Input: part model. Units: mm. Frame: model coordinates. A direction names the side the tool comes from. Give positions to 0.01 mm unless a question says otherwise; leave off trailing zeros. Loops run counter-clockwise (first coordinate to the right, second up) from the corner with the lowest first, then second, coordinate; pieces in that order, holes last. Notation, with made-up numbers: M 57.25,69 L 76.25,69 A32 ccw 76.25,100 Z; hole C 67.5,-7.75 d11. An arc over 180 degrees is marked long. Use a Markdown table: item, result. Add a question column.
Autodesk Inventor part; units mm, degrees
ref_plane "YZ Plane" through (0, 0, 0) normal (1, 0, 0) x (0, 1, 0)
ref_plane "XZ Plane" through (0, 0, 0) normal (0, 1, 0) x (-1, 0, 0)
ref_plane "XY Plane" through (0, 0, 0) normal (0, 0, 1) x (1, 0, 0)
sketch "Szkic1" plane through (0, 0, 0) normal (0, 1, 0) x (-1, 0, 0)
  line L0 (0, 0) -> (25, 0)
  line L1 (25, 0) -> (25, -25)
  line L2 (25, -25) -> (0, -25)
  line L3 (0, -25) -> (0, 0)
  line L4 (25, -5) -> (31, -5)
  line L5 (31, -5) -> (31, -20)
  line L6 (31, -20) -> (25, -20)
  line L7 (25, -20) -> (25, -5)
  circle A0 centre (7.5, -7.5) radius 2.6
  circle A1 centre (7.5, -17.5) radius 2.6
  line L8 (25, -12.5) -> (0, -12.5) construction
  line L9 (18.4, -18) -> (15.4, -18)
  line L10 (15.4, -18) -> (15.4, -7)
  line L11 (15.4, -7) -> (18.4, -7)
  line L12 (18.4, -7) -> (18.4, -18)
  dimension "d0" = 5.2
  dimension "d1" = 25
  dimension "d2" = 25
  dimension "d3" = 7.5
  dimension "d4" = 10
  dimension "d5" = 6
  dimension "d6" = 15
  dimension "d10" = 18.4
  dimension "d11" = 11
  dimension "d12" = 3
extrude "Wyciągnięcie proste1" add sketch "Szkic1" along normal blind 2
fillet "Zaokrąglenie1" radius 2 8 edges at (0, 1, 0) (0, 1, -25) (-25, 1, 0) (-25, 1, -5) (-31, 1, -5) (-31, 1, -20) (-25, 1, -20) (-25, 1, -25)
fillet "Zaokrąglenie2" radius 0.8 4 edges at (-18.4, 1, -18) (-15.4, 1, -18) (-18.4, 1, -7) (-15.4, 1, -7)
properties part number "pokrywka" material "PLA"
1) Section query C-C, the plane z = -13.25. Return the cut outline in (x, y), and give its area (3 significant figures).
2) Section query B-B, the plane z = -16.5. Return the cut outline in (x, y).
3) Section query A-A, the plane x = -6.5. Return the cut outline in (y, z), and give its area (3 significant figures).
4) Contact query for flat-ended pins moving along their axis: P1, Ø0.8, axis at y = 0.5, z = -2.5, coming from the -X side; P2, Ø1, axis at x = -27.5, y = 1.5, coming from the -Z side. Output: stop coordinate, or through.
5) Section query D-D, the plane x = -26. Return the cut outline in (y, z), and give its area (3 significant figures).
6) Ray query, line 1 (Z direction, x = -7.5, y = 1.25); line 2 (X direction, y = 1.1, z = -11.5); line 3 (X direction, y = 1.9, z = -16.5). Return the intervals inside material, ascending. Write a range as [from, to].
7) Pull-direction query (Z, two-part tool) for faces 1 (the flat face through (-25, 1, -2.5)), 2 (the flat face through (-18.4, 1, -12)), 3 (the flat face through (-28, 1, -20)); classes: pulls with the +Z half, pulls with the -Z half, needs draft (parallel to the pull), parting line crosses it, or undercut.
8) Reachability of faces 4 (the cylindrical face through (-18.17, 1.01, -7.24)), 5 (the flat face through (-25, 1, -22.5)), 6 (the flat face through (-28, 1, -5)), 7 (the flat face through (-31, 1, -12)) from +Z, -Z, +X, -X, +Y, -Y: full face, straight path, thin tool, end or side. Return the list, or none.
Entries:
| question | item | result |
|---|---|---|
| 1 | outline | M -31,0 L -18.4,0 L -18.4,2 L -31,2 Z; M -15.4,0 L 0,0 L 0,2 L -15.4,2 Z |
| 1 | area | 56.0 mm² |
| 2 | outline | M -31,0 L -18.4,0 L -18.4,2 L -31,2 Z; M -15.4,0 L -9.9,0 L -9.9,2 L -15.4,2 Z; M -5.1,0 L 0,0 L 0,2 L -5.1,2 Z |
| 3 | outline | M 0,-25 L 2,-25 L 2,-19.9 L 0,-19.9 Z; M 0,-15.1 L 2,-15.1 L 2,-9.9 L 0,-9.9 Z; M 0,-5.1 L 2,-5.1 L 2,0 L 0,0 Z |
| 3 | area | 30.8 mm² |
| 4 | P1 | stops at x = -25 |
| 4 | P2 | stops at z = -20 |
| 5 | outline | M 0,-20.27 L 2,-20.27 L 2,-4.73 L 0,-4.73 Z |
| 5 | area | 31.1 mm² |
| 6 | line 1 | z = [-25, -20.1], [-14.9, -10.1], [-4.9, 0] |
| 6 | line 2 | x = [-31, -18.4], [-15.4, 0] |
| 6 | line 3 | x = [-31, -18.4], [-15.4, -9.9], [-5.1, 0] |
| 7 | face 1 | needs draft |
| 7 | face 2 | undercut |
| 7 | face 3 | pulls with the -Z half |
| 8 | face 4 | +Y, -Y |
| 8 | face 5 | -Z, -X, +Y, -Y |
| 8 | face 6 | +Z, -X, +Y, -Y |
| 8 | face 7 | +Z, -Z, -X, +Y, -Y |
